Could you check a few things on this model? Use its own coordinates, in mm. Coordinates: 2 decimals unless noted, no trailing zeros. Write each loop counter-clockwise with the first axis right and the second up, starting at its lowest first coordinate (ties: lowest second). Pieces come first, ordered by that corner, then holes. Notation, with made-up numbers: M -27,14 L 23,14 A24 ccw 23,34 Z; hole C -0.5,20.5 d9. An arc over 180 degrees is marked long. Answer as CSV lines item,"result". Start each with the question number.
Item 1: I'm going to push flat-ended pins straight in: P1, Ø2, axis at y = -0.5, z = -72.5, coming from the -X side; P2, Ø1.5, axis at x = -13.5, y = 1, coming from the -Z side; P3, Ø4.5, axis at x = 0, y = 0, coming from the -Z side. Where does each tip first touch, or does it pass through?
Item 2: If I drill on line 1 along Y through (x, z) = (0, -202.2); line 2 along Z through (x, y) = (-28, 1.25); line 3 along X through (y, z) = (0, -201.75), over which ranges is the centre line in solid material (lowest first)? Write a range as [from, to].
Item 3: Suppose I cut it at A-A, the plane z = -126.5. Write out the boundary of the cut face in (x, y).
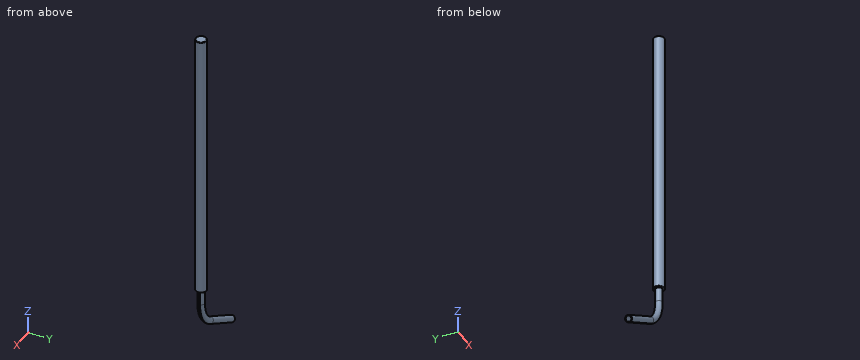
```python
from build123d import *

# Parameters (mm, degrees)
SKETCH1_R      = 3.96875
EXTRUDE1_DEPTH = 200
FILLET1_R      = 0.508


with BuildPart() as part:
    # Sketch1 → Extrude1 (new body)
    with BuildSketch(Plane.XY):
        Circle(SKETCH1_R)
    extrude(amount=-EXTRUDE1_DEPTH)

    # Fillet1
    fillet1_edges = [part.edges().sort_by_distance(p)[0] for p in [
        (-3.96875, 0, 0),
        (-3.96875, 0, -200),
    ]]
    fillet(fillet1_edges, radius=FILLET1_R)

    # Sweep1: sweep along a path in Sketch2
    with BuildLine(Plane(origin=(0, 0, 0), x_dir=(1, 0, 0), z_dir=(0, 1, 0))) as sweep1_path:
        Line((0, 200), (0, 210.56624327))
        ThreePointArc((0, 210.56624327), (-3.349364905, 223.06624327), (-12.5, 232.216878365))
        Line((-12.5, 232.216878365), (-43.301270189, 250))
    # Sketch3 → Sweep1 (sweep)
    with BuildSketch(Plane(origin=(0, 0, -200), x_dir=(-1, 0, 0), z_dir=(0, 0, -1))):
        with BuildLine():
            Line((-2.449489743, 0.5), (-1.936491673, 0.5))
            ThreePointArc((-1.936491673, 0.5), (2, 0), (-1.936491673, -0.5))
            Line((-1.936491673, -0.5), (-2.449489743, -0.5))
            ThreePointArc((-2.449489743, -0.5), (2.5, 0), (-2.449489743, 0.5))
        make_face()
    sweep(path=sweep1_path.line)

    # Sketch4 → Cut-Revolve3 (revolve, cut)
    with BuildSketch(Plane(origin=(0, 0, -205), x_dir=(-1, 0, 0), z_dir=(0, 0, -1))):
        with BuildLine():
            Line((0, 2.25), (0, -2.25))
            ThreePointArc((0, -2.25), (2.25, 0), (0, 2.25))
        make_face()
    revolve(axis=Axis((0, 0, -205), (0, 1, 0)), mode=Mode.SUBTRACT)


solid = part.part
```
Ans:
1,P1,"stops at x = -3.97"
1,P2,"stops at z = -235.96"
1,P3,"stops at z = -225.84"
2,line 1,"y = [-2.5, -2], [2, 2.5]"
2,line 2,"z = [-243.67, -242.97], [-239.36, -238.67]"
2,line 3,"x = [-2.5, -2]"
3,outline,"C 0,0 d7.94"
